Verification items for the finished model (mm, model axes). Face numbers are marked on the shaded views. Coordinates: 2 decimals unless noted, no trailing zeros. Write each loop counter-clockwise with the first axis right and the second up, starting at its lowest first coordinate (ties: lowest second). Pieces come first, ordered by that corner, then holes. Notation, with made-up numbers: (58.5, -30.75) - (84.5, -30.75) arc R12 cw to (84.5, -7.75) - close; hole circle Ø11 at (19, -11.75). An arc over 180 degrees is marked (long way). Use CSV: the item, a comma, the result in double quotes. Start each with the question number.
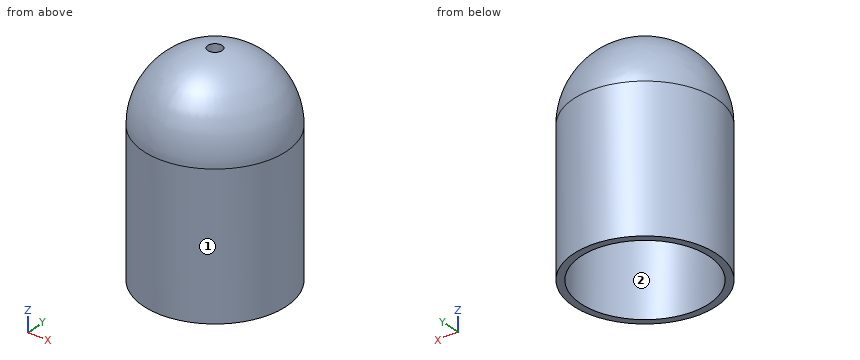
```python
from build123d import *

# Parameters (mm, degrees)
F2_R     = 45
F3_DEPTH = 100
F4_R     = 5
F5_DEPTH = 150.001


with BuildPart() as f1:
    # F0 (on Front) → F1 (revolve)
    with BuildSketch(Plane.XZ):
        with BuildLine():
            Line((-50, 0), (0, 0))
            Line((0, 0), (0, 150))
            ThreePointArc((0, 150), (-35.355339, 135.355339), (-50, 100))
            Line((-50, 100), (-50, 0))
        make_face()
    revolve(axis=Axis((0, 0, 75), (0, 0, 1)))

    # F2 (on Top) → F3 (cut)
    with BuildSketch(Plane.XY):
        Circle(F2_R)
    extrude(amount=F3_DEPTH, mode=Mode.SUBTRACT)

    # F4 (on Top) → F5 (cut, through all)
    with BuildSketch(Plane.XY):
        Circle(F4_R)
    extrude(amount=F5_DEPTH, mode=Mode.SUBTRACT)


solid = f1.part
```
Q1. Cross-section at A-A (z = 28). Record the cut outline in (x, y), plus the area to 3 significant figures.
Q2. Scan lines: line 1 along Y through (x, z) = (0, 71); line 2 along X through (y, z) = (-31, 65); line 3 along X through (y, z) = (-27, 18). Record each from-to range of solid material in increasing order. Write a range as from..to.
Q3. Release check for a two-part mould opening along Y. For the marked faces 1 and 2 record: released by +Y, released by -Y, zero draft, split by the parting line, or undercut.
Q4. Gauge pin test, flat ends, axial feed: pin 1 (1 mm diameter, centred on x = -17.5, z = 109.5, fed in from +Y); pin 2 (4 mm diameter, centred on x = 1.5, z = 123.5, fed in from -Y); pin 3 (1 mm diameter, centred on x = 9.5, y = 11, fed in from +Z). Record the tip position at first contact, or that the pin passes through.
Reply:
1,outline,"circle Ø100 at (0, 0); hole circle Ø90 at (0, 0)"
1,area,"1,490 mm^2"
2,line 1,"-50..-45, 45..50"
2,line 2,"-39.23..-32.62, 32.62..39.23"
2,line 3,"-42.08..-36, 36..42.08"
3,face 1,"split by the parting line"
3,face 2,"undercut"
4,pin 1,"y = 46.08"
4,pin 2,"y = -45.12"
4,pin 3,"z = 147.99"
